The listing builds one solid part. Answer for the finished solid, in the listing's coordinates (mm). Face numbers are marked on the shaded views. Give positions to 0.01 mm unless a question says otherwise; leave off trailing zeros. Loops run counter-clockwise (first coordinate to the right, second up) from the corner with the lowest first, then second, coordinate; pieces in that order, holes last. Notation, with made-up numbers: (3.25, 59) - (22.25, 59) arc R14 ccw to (22.25, 73) - close; hole circle Ø4 at (21, 24). An arc over 180 degrees is marked (long way). Answer in a Markdown table with one row per item. Add a question column.
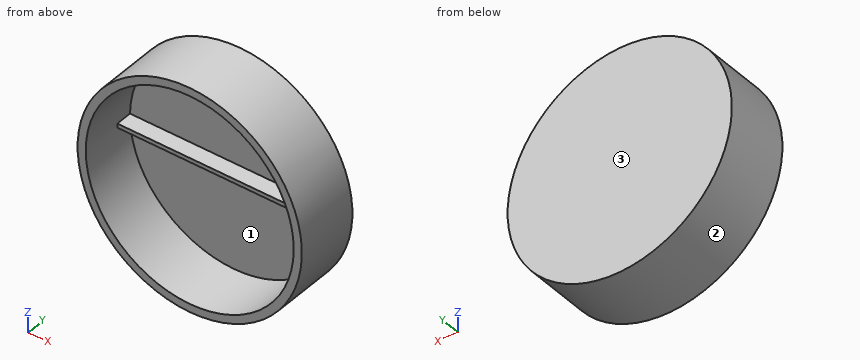
```python
from build123d import *

# Parameters (mm, degrees)
SKETCH2_W           = 81.026
SKETCH2_H           = 1.5875
BOSS_EXTRUDE1_DEPTH = 6.35


with BuildPart() as part:
    # Sketch1 → Revolve1 (revolve)
    with BuildSketch(Plane.XY, mode=Mode.PRIVATE) as revolve1_sk:
        Polygon((0, 0), (43.688, 0), (43.688, -25.4), (40.513, -25.4), (40.513, -3.175), (0, -3.175), align=None)
    revolve(revolve1_sk.sketch.rotate(Axis((0, -3.175, 0), (0, 1, 0)), 90), axis=Axis((0, -3.175, 0), (0, 1, 0)))

    # Sketch2 → Boss-Extrude1 (add)
    with BuildSketch(Plane.XZ.offset(3.175)):
        Rectangle(SKETCH2_W, SKETCH2_H)
    extrude(amount=BOSS_EXTRUDE1_DEPTH)


solid = part.part
```
(1) A cutting plane is placed at B-B on x = 0. Determine the outline of the cut face in (y, z) (3 decimals), plus the area to 3 significant figures.
(2) Given pin 1 Ø2 at (y, z) = (-13.5, 31) entering from +X; pin 2 Ø20 at (x, z) = (19, 12.5) entering from -Y (3 decimals); pin 3 Ø0.5 at (x, z) = (18, 0) entering from -Y (3 decimals), each flat-ended and moving along its own axis, determine where each tip first touches the part or whether it passes through.
(3) The mould has two halves that part along X. Classify the marked faces 1, 2 and 3: pulls with the +X half, pulls with the -X half, needs draft (parallel to the pull), parting line crosses it, or undercut.
(4) Find the intervals of material crossed by line 1 along X through (y, z) = (-14.25, 0); line 2 along Z through (x, y) = (-29, -6.5); line 3 along Z through (x, y) = (-18, -8), in increasing order. Write a range as [from, to].
(5) A cutting plane is placed at D-D on z = 13.5. Determine the outline of the cut face in (x, y) (3 decimals).
(6) A cutting plane is placed at C-C on y = -17.5. Determine the outline of the cut face in (x, z).
Evaluation:
| question | item | result |
|---|---|---|
| 1 | outline | (-25.4, -43.688) - (0, -43.688) - (0, 43.688) - (-25.4, 43.688) - (-25.4, 40.513) - (-3.175, 40.513) - (-3.175, 0.794) - (-9.525, 0.794) - (-9.525, -0.794) - (-3.175, -0.794) - (-3.175, -40.513) - (-25.4, -40.513) - close |
| 1 | area | 429 mm² |
| 2 | pin 1 | stops at x = 31.76 |
| 2 | pin 2 | stops at y = -3.175 |
| 2 | pin 3 | stops at y = -9.525 |
| 3 | face 1 | undercut |
| 3 | face 2 | parting line crosses it |
| 3 | face 3 | needs draft |
| 4 | line 1 | x = [-43.69, -40.51], [40.51, 43.69] |
| 4 | line 2 | z = [-32.67, -28.29], [-0.79, 0.79], [28.29, 32.67] |
| 4 | line 3 | z = [-39.81, -36.29], [-0.79, 0.79], [36.29, 39.81] |
| 5 | outline | (-41.55, -25.4) - (-38.198, -25.4) - (-38.198, -3.175) - (38.198, -3.175) - (38.198, -25.4) - (41.55, -25.4) - (41.55, 0) - (-41.55, 0) - close |
| 6 | outline | circle Ø87.38 at (0, 0); hole circle Ø81.03 at (0, 0) |
